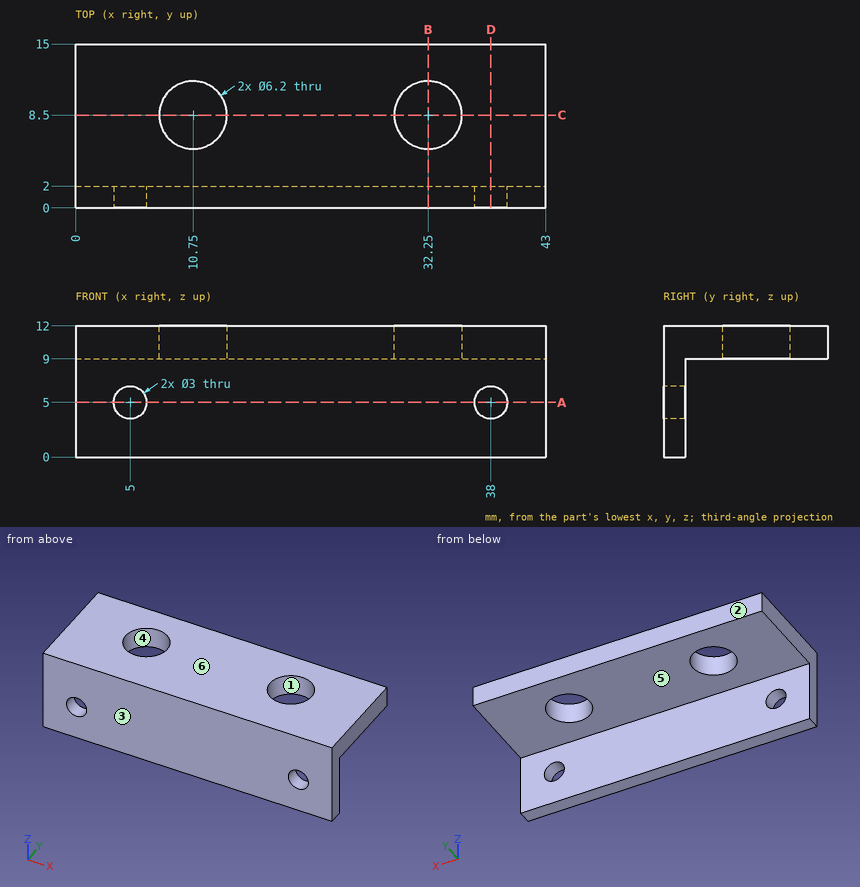
Check sheet for the drawn part. Datum: minimum x, y, z corner. Units: mm. A direction names the side the tool comes from. Coordinates: 2 decimals unless noted, no trailing zeros. Loops run counter-clockwise (first coordinate to the right, second up) from the corner with the lowest first, then second, coordinate; pieces in that order, holes last. Notation, with made-up numbers: (89, 58) -> (101, 58) arc R26 ccw to (101, 85) -> close; hole circle Ø4 at (38.25, 13.25). An arc over 180 degrees is marked (long way). Answer in a Markdown table with one row per item.
1. Material ranges on line 1 along X through (y, z) = (1.25, 5); line 2 along Z through (x, y) = (5, 1); line 3 along X through (y, z) = (7, 10.75), recorded low to high. Write a range as [from, to].
Check values:
| item | result |
|---|---|
| line 1 | x = [0, 3.5], [6.5, 36.5], [39.5, 43] |
| line 2 | z = [0, 3.5], [6.5, 12] |
| line 3 | x = [0, 8.04], [13.46, 29.54], [34.96, 43] |
2. Sectioned sample at C-C, the plane y = 8.5. Record the boundary of the cut face in (x, z), then the cut area to 3 significant figures.
Check values:
| item | result |
|---|---|
| outline | (0, 9) -> (7.65, 9) -> (7.65, 12) -> (0, 12) -> close; (13.85, 9) -> (29.15, 9) -> (29.15, 12) -> (13.85, 12) -> close; (35.35, 9) -> (43, 9) -> (43, 12) -> (35.35, 12) -> close |
| area | 91.8 mm2 |
3. Sectioned sample at D-D, the plane x = 38. Record the boundary of the cut face in (y, z).
Check values:
| item | result |
|---|---|
| outline | (0, 0) -> (2, 0) -> (2, 3.5) -> (0, 3.5) -> close; (0, 6.5) -> (2, 6.5) -> (2, 9) -> (15, 9) -> (15, 12) -> (0, 12) -> close |
4. Go/stop test with flat-tipped pins: pin 1 (3 mm diameter, centred on x = 19.5, y = 4.5, fed in from -Z); pin 2 (6 mm diameter, centred on x = 6.5, z = 3.5, fed in from +Y). Record where each tip stops, or that it passes through.
Check values:
| item | result |
|---|---|
| pin 1 | stops at z = 9 |
| pin 2 | stops at y = 2 |
5. Access from +Z, -Z, +X, -X, +Y, -Y to the whole of each face (thin tool, end or side, straight path). Record for the marked faces 5 and 6.
Check values:
| item | result |
|---|---|
| face 5 | -Z, +X, -X, +Y |
| face 6 | +Z, +X, -X, +Y, -Y |
6. Sectioned sample at B-B, the plane x = 32.25. Record the boundary of the cut face in (y, z), then the cut area to 3 significant figures.
Check values:
| item | result |
|---|---|
| outline | (0, 0) -> (2, 0) -> (2, 9) -> (5.4, 9) -> (5.4, 12) -> (0, 12) -> close; (11.6, 9) -> (15, 9) -> (15, 12) -> (11.6, 12) -> close |
| area | 44.4 mm2 |
7. Sectioned sample at A-A, the plane z = 5. Record the boundary of the cut face in (x, y), then the cut area to 3 significant figures.
Check values:
| item | result |
|---|---|
| outline | (0, 0) -> (3.5, 0) -> (3.5, 2) -> (0, 2) -> close; (6.5, 0) -> (36.5, 0) -> (36.5, 2) -> (6.5, 2) -> close; (39.5, 0) -> (43, 0) -> (43, 2) -> (39.5, 2) -> close |
| area | 74.0 mm2 |
8. Release check for a two-part mould opening along Y. For the marked faces 1, 2, 3 and 4 record: released by +Y, released by -Y, zero draft, split by the parting line, or undercut.
Check values:
| item | result |
|---|---|
| face 1 | undercut |
| face 2 | released by +Y |
| face 3 | released by -Y |
| face 4 | undercut |
